Could you check a few things on this model? Use its own coordinates, in mm. Face numbers are marked on the shaded views. A direction names the side the tool comes from. Round coordinates to 2 decimals unless told otherwise and drop trailing zeros. Loops run counter-clockwise (first coordinate to the right, second up) from the corner with the lowest first, then second, coordinate; pieces in that order, holes last. Notation, with made-up numbers: (-6, -38) - (19, -38) arc R9 ccw to (19, -25) - close; hole circle Ø9 at (-10, 87). An arc over 180 degrees is marked (long way). Answer as CSV lines item,"result". Start each with the question number.
1) Please list where these lines run through material, in increasing order: line 1 along X through (y, z) = (0, 11); line 2 along Y through (x, z) = (0, 9.5) (3 decimals); line 3 along Y through (x, z) = (-6, 13.5).
2) Suppose I cut it at C-C, the plane y = 1.5. Write out the boundary of the cut face in (x, z).
3) Suppose I cut it at B-B, the plane z = 13.75. Write out the boundary of the cut face in (x, y) (1 decimal).
4) I'm going to push flat-ended pins straight in: pin 1 Ø1 at (x, z) = (5, 14.5) entering from -Y; pin 2 Ø4 at (x, y) = (-0.5, 3.5) entering from -Z; pin 3 Ø1 at (x, z) = (-4.5, 12.5) entering from +Y; pin 4 Ø1 at (y, z) = (-4, 6) entering from -X. Where does each tip first touch, or does it pass through?
5) Suppose I cut it at A-A, the plane x = 0. Write out the boundary of the cut face in (y, z) (3 decimals).
6) We'd pull the mould along X, two halves only. Please class the marked faces 5, 6 and 7: pulls with the +X half, pulls with the -X half, needs draft (parallel to the pull), parting line crosses it, or undercut.
7) Which directions (+Z, -Z, +X, -X, +Y, -Y) give clear straight access to the entire face, cutting with the end or side of a thin tool? Please do the marked faces 1, 2, 3 and 4.
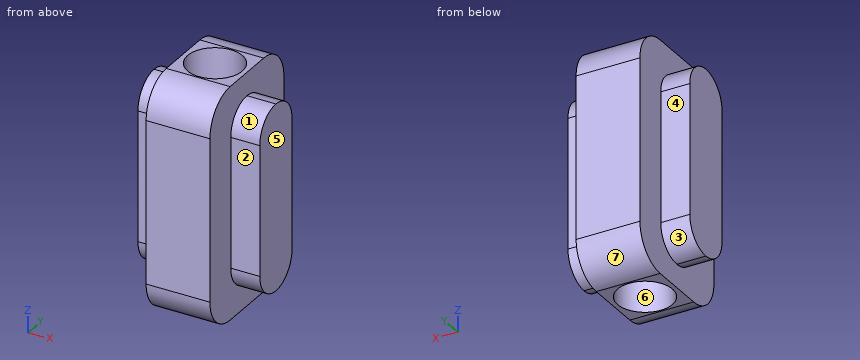
```python
from build123d import *

# Parameters (mm, degrees)
F0_W     = 6.985
F0_H     = 13.97
F1_DEPTH = 25.4
F2_R     = 3
F3_DEPTH = 25.4
F4_W     = 3.048
F4_H     = 20.32
F5_DEPTH = 3.175
F6_R     = 3.04799
F8_R     = 3.81


# Not quite as in the source:
# - a fillet or chamfer is up to 0.001 mm smaller than in the source, because OpenCascade refuses the exact size


with BuildPart() as f1:
    # F0 (on Top) → F1 (new body)
    with BuildSketch(Plane.XY):
        Rectangle(F0_W, F0_H)
    extrude(amount=F1_DEPTH)

    # F2 (on face) → F3 (cut)
    with BuildSketch(Plane(origin=(0, 0, 0), x_dir=(1, 0, 0), z_dir=(0, 0, -1))):
        Circle(F2_R)
    extrude(amount=-F3_DEPTH, mode=Mode.SUBTRACT)

    # F4 (on face) → F5 (join)
    with BuildSketch(Plane.YZ.offset(3.4925)):
        with Locations((1.524, 12.7)):
            Rectangle(F4_W, F4_H)
        with Locations((-1.524, 12.7)):
            Rectangle(F4_W, F4_H)
    extrude(amount=F5_DEPTH)

    # F6 (radius 3.048 in the source; OpenCascade refuses exactly that, so slightly less here)
    f6_edges = [f1.edges().sort_by_distance(p)[0] for p in [
        (5.08, -3.048, 22.86),
        (5.08, 3.048, 22.86),
        (5.08, 3.048, 2.54),
        (5.08, -3.048, 2.54),
    ]]
    fillet(f6_edges, radius=F6_R)

    # F7: F1 across plane


with BuildPart() as f1_1:
    add(f1.part)
    add(f1.part.mirror(Plane.YZ))

    # F8
    f8_edges = [f1_1.edges().sort_by_distance(p)[0] for p in [
        (0, -6.985, 0),
        (0, 6.985, 0),
        (0, 6.985, 25.4),
        (0, -6.985, 25.4),
    ]]
    fillet(f8_edges, radius=F8_R)


solid = f1_1.part
```
Filled sheet:
1,line 1,"-6.67 to -3, 3 to 6.67"
1,line 2,"-6.985 to -3, 3 to 6.985"
1,line 3,"-3.05 to 3.05"
2,outline,"(-6.67, 2.93) - (-3.49, 2.93) - (-3.49, 0) - (-2.6, 0) - (-2.6, 25.4) - (-3.49, 25.4) - (-3.49, 22.47) - (-6.67, 22.47) - close; (2.6, 0) - (3.49, 0) - (3.49, 2.93) - (6.67, 2.93) - (6.67, 22.47) - (3.49, 22.47) - (3.49, 25.4) - (2.6, 25.4) - close"
3,outline,"(-6.7, -3) - (-3.5, -3) - (-3.5, -7) - (3.5, -7) - (3.5, -3) - (6.7, -3) - (6.7, 3) - (3.5, 3) - (3.5, 7) - (-3.5, 7) - (-3.5, 3) - (-6.7, 3) - close; hole circle Ø6 at (0, 0)"
4,pin 1,"y = -3.05"
4,pin 2,"z = 0"
4,pin 3,"y = 3.05"
4,pin 4,"x = -3.49"
5,outline,"(-6.985, 3.81) arc R3.81 ccw to (-3.175, 0) - (-3, 0) - (-3, 25.4) - (-3.175, 25.4) arc R3.81 ccw to (-6.985, 21.59) - close; (3, 0) - (3.175, 0) arc R3.81 ccw to (6.985, 3.81) - (6.985, 21.59) arc R3.81 ccw to (3.175, 25.4) - (3, 25.4) - close"
6,face 5,"pulls with the +X half"
6,face 6,"undercut"
6,face 7,"needs draft"
7,face 1,"+Z, +X, -Y"
7,face 2,"+Z, -Z, +X, -Y"
7,face 3,"-Z, -X, +Y"
7,face 4,"+Z, -Z, -X, +Y"
